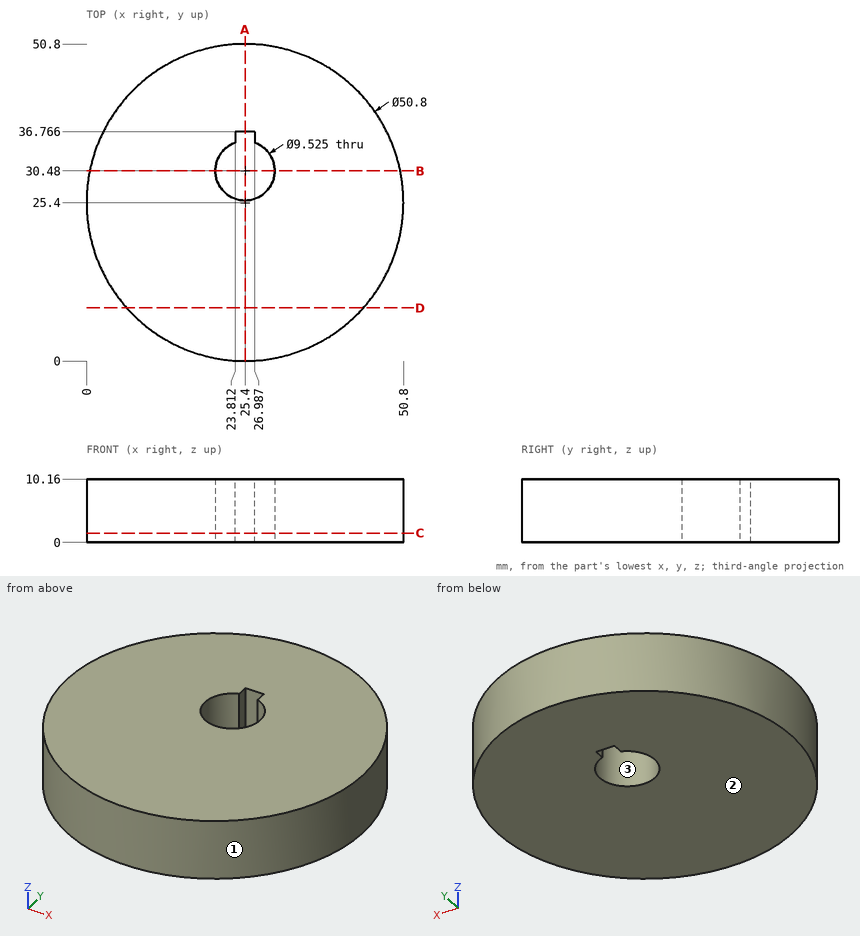
Print and shaded views of the part. All mm, measured from the part's lowest x, y and z. Coordinates: 2 decimals unless noted, no trailing zeros. Loops run counter-clockwise (first coordinate to the right, second up) from the corner with the lowest first, then second, coordinate; pieces in that order, holes last. Notation, with made-up numbers: M 66,30 L 124,30 A28 cw 124,63 Z; hole C 44.25,37 d3. An arc over 180 degrees is marked long. Use a Markdown table: item, result. Add a question column.
Q1. Cut at B-B (y = 30.48). Write the cut outline in (x, z), and give its area (3 significant figures).
Q2. Pin check, flat tips, straight feed: P1, Ø0.5, axis at y = 36.5, z = 3, coming from the -X side (1 decimal); P2, Ø3, axis at y = 30.5, z = 8, coming from the -X side; P3, Ø3, axis at x = 20, z = 8, coming from the -Y side. Stop position of each tip, or through.
Q3. Cut at D-D (y = 8.5). Write the cut outline in (x, z).
Q4. Mould opens along Y. For the marked faces 1, 2 and 3 say: +Y half, -Y half, draft (parallel to the pull), parting line (faces both ways), or undercut.
Q5. Cut at C-C (z = 1.5). Write the cut outline in (x, y) (1 decimal).
Q6. Probe L1, parallel to Y at x = 25.4, z = 8.25; L2, parallel to X at y = 30.48, z = 2.75; L3, parallel to Y at x = 27.5, z = 2.5 (1 decimal). List the from-to ranges inside material, lowest first.
Q7. Cut at A-A (x = 25.4). Write the cut outline in (y, z).
Worked out:
| question | item | result |
|---|---|---|
| 1 | outline | M 0.51,0 L 20.64,0 L 20.64,10.16 L 0.51,10.16 Z; M 30.16,0 L 50.29,0 L 50.29,10.16 L 30.16,10.16 Z |
| 1 | area | 409 mm2 |
| 2 | P1 | stops at x = 2.4 |
| 2 | P2 | stops at x = 0.26 |
| 2 | P3 | stops at y = 0.3 |
| 3 | outline | M 6.44,0 L 44.36,0 L 44.36,10.16 L 6.44,10.16 Z |
| 4 | face 1 | parting line |
| 4 | face 2 | draft |
| 4 | face 3 | undercut |
| 5 | outline | C 25.4,25.4 d50.8; hole M 23.8,35 A4.8 ccw long 27,35 L 27,36.8 L 23.8,36.8 Z |
| 6 | L1 | y = 0 to 25.72, 36.77 to 50.8 |
| 6 | L2 | x = 0.51 to 20.64, 30.16 to 50.29 |
| 6 | L3 | y = 0.1 to 26.2, 34.8 to 50.7 |
| 7 | outline | M 0,0 L 25.72,0 L 25.72,10.16 L 0,10.16 Z; M 36.77,0 L 50.8,0 L 50.8,10.16 L 36.77,10.16 Z |
